For this review, take the finished solid that the model builds, in its own axes (mm). A direction names the side the tool comes from. Coordinates: 2 decimals unless noted, no trailing zeros. Write each loop counter-clockwise with the first axis right and the second up, starting at its lowest first coordinate (ties: lowest second). Pieces come first, ordered by that corner, then holes. Notation, with made-up numbers: (21, 42.5) -> (65, 42.5) arc R30 ccw to (65, 65.5) -> close; hole circle Ø7 at (-18.5, -20). An arc over 180 degrees is marked (long way). One line per item, written item: value. Start each with the question number.
1) Add section C-C (z = -10.5). State the section outline as (x, y) points, and give its area (3 significant figures).
2) For pin 1 Ø2.5 at (x, y) = (37.5, -4) entering from +Z; pin 2 Ø3 at (x, y) = (-14.5, -9) entering from +Z; pin 3 Ø3.5 at (x, y) = (20, -12.5) entering from +Z, all flat-tipped, find the tip position at first contact; note any pin that passes through.
3) For probe 1 along X at (y, z) = (-12.95, -0.5); probe 2 along X at (y, z) = (-6.5, -6); probe 3 along Y at (x, z) = (-37, -6.35), list the stretches that pass through material, from the lowest coordinate up. Write a range as from..to.
4) Mouldability with a two-part tool opening along Z and no side actions: class faces 1 (the flat face through (37, -4, -7.5)), 2 (the cylindrical face through (-38.65, -12.48, -0.43)), 3 (the flat face through (5, -11, 8)) as released by +Z, released by -Z, zero draft, split by the parting line, or undercut.
5) Add section A-A (z = -0.5). State the section outline as (x, y) points, and give its area (3 significant figures).
6) Machinability: for faces 4 (the flat face through (-21, -12, 4.5)), 5 (the flat face through (-34, -7, -10)), 6 (the flat face through (-30, -10, -1)), 7 (the flat face through (-18, -10, 2.5)), which of the approach directions +Z, -Z, +X, -X, +Y, -Y give a long, thin tool a straight path to every point of the face, cutting with its end or side? Answer none if there is none.
7) Add section B-B (y = -7.75). State the section outline as (x, z) points.
8) Add section D-D (x = 28). State the section outline as (y, z) points, and give its area (3 significant figures).
from build123d import *

# Parameters (mm, degrees)
F0_R      = 1.65
F1_DEPTH  = 14
F2_W      = 11
F2_H      = 9
F3_DEPTH  = 80.001
F4_R      = 1.3
F5_DEPTH  = 80.001
F6_R      = 3
F7_SIZE   = 2
F8_R      = 1.5
F9_DEPTH  = 3
F11_DEPTH = 2.5
F12_W     = 10
F12_H     = 8
F12_H_2   = 2
F13_DEPTH = 5.5
F14_R     = 2.5
F15_R     = 1.3
F16_DEPTH = 45.001


with BuildPart() as f1:
    # F0 (on Front) → F1 (new body)
    with BuildSketch(Plane.XZ):
        Polygon((-34, -4.5), (34, -4.5), (34, -14.5), (40, -14.5), (40, -4.5), (40, 4.5), (-40, 4.5), (-40, -4.5), (-40, -14.5), (-34, -14.5), align=None)
        with Locations((-37, -0.5)):
            Circle(F0_R, mode=Mode.SUBTRACT)
        with Locations((37, -0.5)):
            Circle(F0_R, mode=Mode.SUBTRACT)
    extrude(amount=F1_DEPTH)

    # F2 (on face) → F3 (cut, through all)
    with BuildSketch(Plane.YZ.offset(40)):
        with Locations((-5.5, 0)):
            Rectangle(F2_W, F2_H)
    extrude(amount=-F3_DEPTH, mode=Mode.SUBTRACT)

    # F4 (on face) → F5 (cut, through all)
    with BuildSketch(Plane.YZ.offset(40)):
        with Locations((-10, -10.5)):
            Circle(F4_R)
    extrude(amount=-F5_DEPTH, mode=Mode.SUBTRACT)

    # F6
    f6_edges = [f1.edges().sort_by_distance(p)[0] for p in [
        (37, -14, -14.5),
        (-37, -14, -14.5),
        (-37, 0, -14.5),
        (37, 0, -14.5),
        (40, -12.5, 4.5),
        (-40, -12.5, 4.5),
    ]]
    fillet(f6_edges, radius=F6_R)

    # F7
    f7_edges = [f1.edges().sort_by_distance(p)[0] for p in [
        (34, -12.5, -4.5),
        (-34, -12.5, -4.5),
    ]]
    chamfer(f7_edges, length=F7_SIZE)

    # F8 (on face) → F9 (cut)
    with BuildSketch(Plane.XY.offset(-4.5)):
        with Locations((-37, -3.75)):
            Circle(F8_R)
        with Locations((37, -3.75)):
            Circle(F8_R)
    extrude(amount=-F9_DEPTH, mode=Mode.SUBTRACT)

    # F10 (on face) → F11 (join)
    with BuildSketch(Plane(origin=(0, -11, 0), x_dir=(-1, 0, 0), z_dir=(0, 1, 0))):
        Polygon((-5, 2.5), (-30, 2.5), (-30, -4.5), (30, -4.5), (30, 2.5), (5, 2.5), (5, 4.5), (-5, 4.5), align=None)
    extrude(amount=F11_DEPTH)

    # F12 (on face) → F13 (join)
    with BuildSketch(Plane(origin=(0, -8.5, 0), x_dir=(-1, 0, 0), z_dir=(0, 1, 0))):
        with Locations((0, 8.5)):
            Rectangle(F12_W, F12_H)
        with Locations((0, 3.5)):
            Rectangle(F12_W, F12_H_2)
    extrude(amount=-F13_DEPTH)

    # F14
    f14_edges = [f1.edges().sort_by_distance(p)[0] for p in [
        (0, -14, 12.5),
        (0, -8.5, 12.5),
    ]]
    fillet(f14_edges, radius=F14_R)

    # F15 (on face) → F16 (cut, through all)
    with BuildSketch(Plane.YZ.offset(5)):
        with Locations((-11.25, 9.5)):
            Circle(F15_R)
    extrude(amount=-F16_DEPTH, mode=Mode.SUBTRACT)


solid = f1.part
Numbers:
1. outline: (-40, -14) -> (-34, -14) -> (-34, -11.3) -> (-40, -11.3) -> close; (-40, -8.7) -> (-34, -8.7) -> (-34, 0) -> (-40, 0) -> close; (34, -14) -> (40, -14) -> (40, -11.3) -> (34, -11.3) -> close; (34, -8.7) -> (40, -8.7) -> (40, 0) -> (34, 0) -> close
1. area: 137 mm²
2. pin 1: z = -4.5
2. pin 2: z = 2.5
2. pin 3: z = 4.5
3. probe 1: -40..-38.65, -35.35..35.35, 38.65..40
3. probe 2: -40..-34, 34..40
3. probe 3: -14..-5.25, -2.25..0
4. face 1: released by +Z
4. face 2: undercut
4. face 3: zero draft
5. outline: (-40, -14) -> (-38.65, -14) -> (-38.65, -11) -> (-40, -11) -> close; (-35.35, -14) -> (35.35, -14) -> (35.35, -11) -> (30, -11) -> (30, -8.5) -> (-30, -8.5) -> (-30, -11) -> (-35.35, -11) -> close; (38.65, -14) -> (40, -14) -> (40, -11) -> (38.65, -11) -> close
5. area: 370 mm²
6. face 4: +Z, -X, +Y, -Y
6. face 5: -Z, +Y
6. face 6: +Z, -Z, -X, +Y
6. face 7: +Z, -X, +Y
7. outline: (-40, -14.5) -> (-34, -14.5) -> (-34, -4.5) -> (-40, -4.5) -> close; (34, -14.5) -> (40, -14.5) -> (40, -4.5) -> (34, -4.5) -> close
8. outline: (-14, -4.5) -> (-8.5, -4.5) -> (-8.5, 2.5) -> (-11, 2.5) -> (-11, 4.5) -> (-14, 4.5) -> close
8. area: 44.5 mm²
